Answer from the drawing. Dimensions are ordinates in mm from the lowest x, y and z of the part. Round coordinates to 2 decimals unless told otherwise and drop trailing zeros. Order: outer loops, then holes, each group sorted by start corner. A loop starts at its lowest first (then second) coordinate and runs counter-clockwise, first axis right, second up. Notation, with made-up numbers: M -1.5,31 L 16.5,31 A8 cw 16.5,42 Z; hole C 39,81 d9. An arc over 180 degrees is marked long. Answer as a JSON object with one key per item and string values. Group by question number.
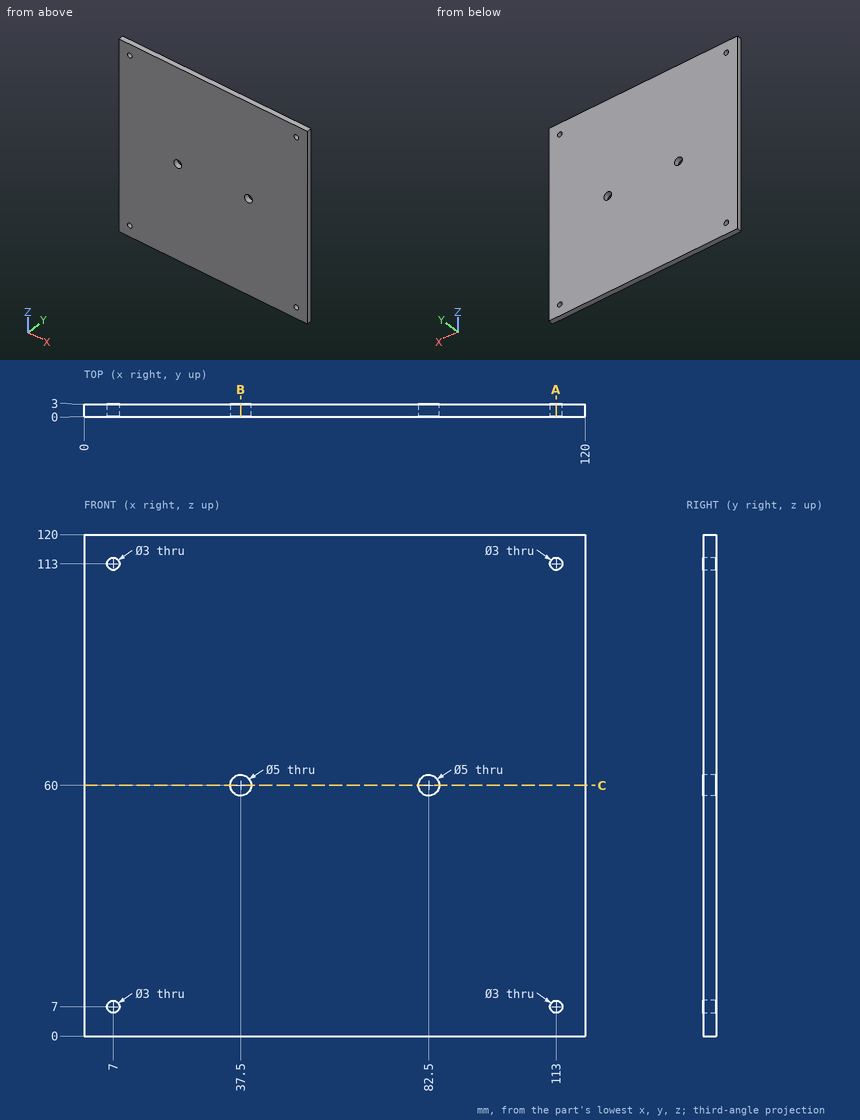
Item 1: Find section A-A (x = 113). Give the vertices of the cut face in (y, z), and give its area (3 significant figures).
Item 2: Consider L1, parallel to X at y = 1.95, z = 113; L2, parallel to X at y = 2.4, z = 60. Determine where each line is inside the solid, lowest interval first.
Item 3: This flat-tipped pin is pushed along its axis until it touches: pin 1 (1.8 mm diameter, centred on x = 113, z = 7, fed in from -Y). Where does it stop, or does it pass through?
Item 4: Find section B-B (x = 37.5). Give the vertices of the cut face in (y, z).
Item 5: Find section C-C (z = 60). Give the vertices of the cut face in (x, y), and give its area (3 significant figures).
Responses:
{
 "1": {"outline": "M 0,0 L 3,0 L 3,5.5 L 0,5.5 Z; M 0,8.5 L 3,8.5 L 3,111.5 L 0,111.5 Z; M 0,114.5 L 3,114.5 L 3,120 L 0,120 Z", "area": "342 mm^2"},
 "2": {"L1": "x = 0 to 5.5, 8.5 to 111.5, 114.5 to 120", "L2": "x = 0 to 35, 40 to 80, 85 to 120"},
 "3": {"pin 1": "passes through"},
 "4": {"outline": "M 0,0 L 3,0 L 3,57.5 L 0,57.5 Z; M 0,62.5 L 3,62.5 L 3,120 L 0,120 Z"},
 "5": {"outline": "M 0,0 L 35,0 L 35,3 L 0,3 Z; M 40,0 L 80,0 L 80,3 L 40,3 Z; M 85,0 L 120,0 L 120,3 L 85,3 Z", "area": "330 mm^2"}
}
